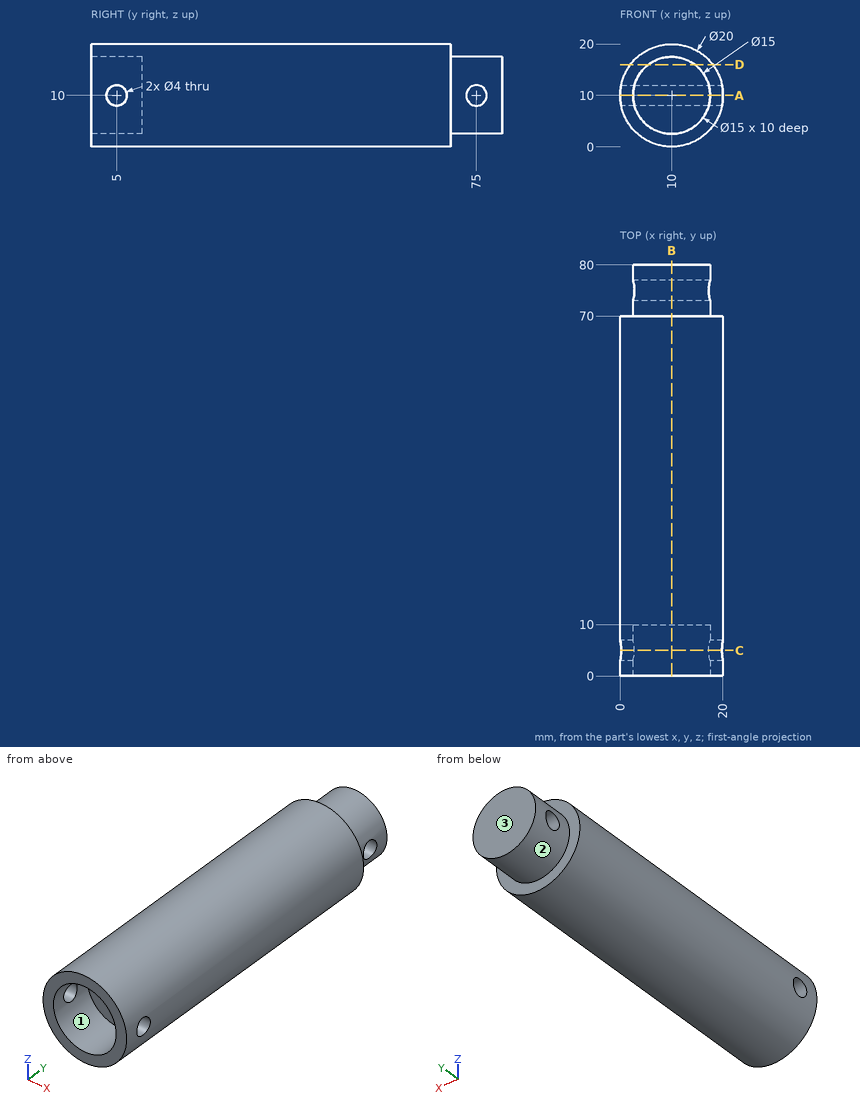
Answer from the drawing. Dimensions are ordinates in mm from the lowest x, y and z of the part. Give positions to 0.01 mm unless a question says otherwise; leave off trailing zeros. Order: outer loops, then holes, each group sorted by start corner. A loop starts at its lowest first (then second) coordinate and runs counter-clockwise, first axis right, second up. Notation, with made-up numbers: (8, -36.5) -> (49, -36.5) arc R18 ccw to (49, -13.5) -> close; hole circle Ø5 at (7, -15.5). An arc over 180 degrees is marked (long way). One line per item, written item: value. Start each with the question number.
(1) The part is cut by section B-B (x = 10). Determine the outline of the cut face in (y, z).
(2) Straight lines are drawn through the part: L1, parallel to Z at x = 10, y = 7.25; L2, parallel to Y at x = 5, z = 1.5; L3, parallel to Y at x = 11.5, z = 12.5. For each, find the intervals that lie inside material, in ascending order.
(3) The part is cut by section D-D (z = 16). Determine the outline of the cut face in (x, y), and give its area (3 significant figures).
(4) Flat-ended cylindrical pins translate along their axes: P1, Ø3.5, axis at y = 5, z = 10, coming from the -X side (3 decimals); P2, Ø1, axis at x = 17, y = 22, coming from the -Z side; P3, Ø8, axis at x = 12, y = 33.5, coming from the +Z side; P4, Ø12, axis at x = 17.5, y = 8, coming from the -Z side. Find the tip coordinate at first contact, or state that the pin passes through.
(5) The part is cut by section A-A (z = 10). Determine the outline of the cut face in (x, y).
(6) The part is cut by section C-C (y = 5). Determine the outline of the cut face in (x, z), and give its area (3 significant figures).
(7) For a pull along Z with two mould halves and no side action, classify the marked faces 1, 2 and 3 as released by +Z, released by -Z, zero draft, split by the parting line, or undercut.
Taken from the geometry:
1. outline: (0, 0) -> (70, 0) -> (70, 2.5) -> (80, 2.5) -> (80, 17.5) -> (70, 17.5) -> (70, 20) -> (0, 20) -> (0, 17.5) -> (10, 17.5) -> (10, 2.5) -> (0, 2.5) -> close; hole circle Ø4 at (75, 10)
2. L1: 0 to 2.5, 17.5 to 20
2. L2: 0 to 70
2. L3: 10 to 80
3. outline: (2, 0) -> (5.5, 0) -> (5.5, 10) -> (14.5, 10) -> (14.5, 0) -> (18, 0) -> (18, 70) -> (14.5, 70) -> (14.5, 80) -> (5.5, 80) -> (5.5, 70) -> (2, 70) -> close
3. area: 1,120 mm^2
4. P1: through
4. P2: z = 2.4
4. P3: z = 20
4. P4: z = 0.11
5. outline: (0, 0) -> (2.5, 0) -> (2.5, 3) -> (0, 3) -> close; (0, 7) -> (2.5, 7) -> (2.5, 10) -> (17.5, 10) -> (17.5, 7) -> (20, 7) -> (20, 70) -> (17.5, 70) -> (17.5, 73) -> (2.5, 73) -> (2.5, 70) -> (0, 70) -> close; (2.5, 77) -> (17.5, 77) -> (17.5, 80) -> (2.5, 80) -> close; (17.5, 0) -> (20, 0) -> (20, 3) -> (17.5, 3) -> close
6. outline: (0.2, 8) arc R10 ccw to (19.8, 8) -> (17.23, 8) arc R7.5 cw to (2.77, 8) -> close; (0.2, 12) -> (2.77, 12) arc R7.5 cw to (17.23, 12) -> (19.8, 12) arc R10 ccw to start
6. area: 117 mm^2
7. face 1: undercut
7. face 2: split by the parting line
7. face 3: zero draft
